```python
from build123d import *

# Parameters (mm, degrees)
SKETCH1_R           = 11.2
BOSS_EXTRUDE1_DEPTH = 50.8
SKETCH2_R           = 3.675
CUT_EXTRUDE1_DEPTH  = 50.8


with BuildPart() as part:
    # Sketch1 → Boss-Extrude1 (new body)
    with BuildSketch(Plane.XY):
        with BuildLine():
            Line((-25.4, -36.364999962), (-25.4, 36.365))
            ThreePointArc((-25.4, 36.365), (-23.726115254, 40.406115254), (-19.685, 42.08))
            Line((-19.685, 42.08), (32.385, 42.08))
            ThreePointArc((32.385, 42.08), (36.426115254, 40.406115254), (38.1, 36.365))
            Line((38.1, 36.365), (38.1, 35.095))
            ThreePointArc((38.1, 35.095), (36.426115254, 31.053884746), (32.385, 29.38))
            Line((32.385, 29.38), (-9.652, 29.38))
            ThreePointArc((-9.652, 29.38), (-11.807261469, 28.487261469), (-12.7, 26.332))
            Line((-12.7, 26.332), (-12.7, 22.503))
            ThreePointArc((-12.7, 22.503), (-11.807261469, 20.347738531), (-9.652, 19.455))
            Line((-9.652, 19.455), (0, 19.455))
            Line((0, 19.455), (13.74, 19.455))
            ThreePointArc((13.74, 19.455), (17.781115254, 17.781115254), (19.455, 13.74))
            Line((19.455, 13.74), (19.455, 0))
            Line((19.455, 0), (19.455, -13.74))
            ThreePointArc((19.455, -13.74), (17.781115254, -17.781115254), (13.74, -19.455))
            Line((13.74, -19.455), (0, -19.455))
            Line((0, -19.455), (-9.652, -19.455))
            ThreePointArc((-9.652, -19.455), (-11.807261469, -20.347738531), (-12.7, -22.503))
            Line((-12.7, -22.503), (-12.7, -26.331999962))
            ThreePointArc((-12.7, -26.331999962), (-11.807261469, -28.487261431), (-9.652, -29.379999962))
            Line((-9.652, -29.379999962), (32.385, -29.379999962))
            ThreePointArc((32.385, -29.379999962), (36.426115254, -31.053884708), (38.1, -35.094999962))
            Line((38.1, -35.094999962), (38.1, -68.114999962))
            ThreePointArc((38.1, -68.114999962), (36.426115254, -72.156115216), (32.385, -73.829999962))
            Line((32.385, -73.829999962), (31.115, -73.829999962))
            ThreePointArc((31.115, -73.829999962), (27.073884746, -72.156115216), (25.4, -68.114999962))
            Line((25.4, -68.114999962), (25.4, -47.794999962))
            ThreePointArc((25.4, -47.794999962), (23.726115254, -43.753884708), (19.685, -42.079999962))
            Line((19.685, -42.079999962), (-19.685, -42.079999962))
            ThreePointArc((-19.685, -42.079999962), (-23.726115254, -40.406115216), (-25.4, -36.364999962))
        make_face()
        Circle(SKETCH1_R, mode=Mode.SUBTRACT)
    extrude(amount=BOSS_EXTRUDE1_DEPTH)

    # Sketch2 → Cut-Extrude1 (cut)
    with BuildSketch(Plane(origin=(25.4, 0, 0), x_dir=(0, 0, -1), z_dir=(1, 0, 0))):
        with Locations((-25.4, -57.954999962)):
            Circle(SKETCH2_R)
    extrude(amount=CUT_EXTRUDE1_DEPTH, mode=Mode.SUBTRACT)


solid = part.part
```
Input: part model. Units: mm. Frame: model coordinates. A direction names the side the tool comes from. Coordinates: 2 decimals unless noted, no trailing zeros. Write each loop counter-clockwise with the first axis right and the second up, starting at its lowest first coordinate (ties: lowest second). Pieces come first, ordered by that corner, then holes. Notation, with made-up numbers: (61.25, -7.75) -> (120.25, -7.75) arc R28 cw to (120.25, 27.25) -> close; hole circle Ø1 at (32.5, 27). An arc over 180 degrees is marked (long way). Write each question's results on one line, items separated by ' | '.
Item 1: Section query D-D on x = 27. Return loops of the section in (y, z) (3 decimals), plus the area to 3 significant figures.
Conclusion:
outline: (-72.081, 0) -> (-29.38, 0) -> (-29.38, 50.8) -> (-72.081, 50.8) -> close; (29.38, 0) -> (42.08, 0) -> (42.08, 50.8) -> (29.38, 50.8) -> close; hole circle Ø7.35 at (-57.955, 25.4) | area: 2,770 mm^2
Item 2: Material intervals for probe 1 along Y at (x, z) = (0, 31) (3 decimals); probe 2 along Y at (x, z) = (5, 29) (3 decimals); probe 3 along Y at (x, z) = (31.25, 25.4), sorted ascending.
Conclusion:
probe 1: y = -42.08 to -29.38, -19.455 to -11.2, 11.2 to 19.455, 29.38 to 42.08 | probe 2: y = -42.08 to -29.38, -19.455 to -10.022, 10.022 to 19.455, 29.38 to 42.08 | probe 3: y = -73.83 to -61.63, -54.28 to -29.38, 29.38 to 42.08
Item 3: Set-up query: faces 4 (the flat face through (-25.4, -1, 25)), 5 (the cylindrical face through (-11.831, -28.463, 25.044)), 6 (the flat face through (0, -42.08, 25)). Return all of +Z, -Z, +X, -X, +Y, -Y with unobstructed straight access to the full face (end or side cutting, diameter ignored); none if empty.
Conclusion:
face 4: +Z, -Z, -X, +Y, -Y | face 5: +Z, -Z, +X | face 6: +Z, -Z, -X, -Y
Item 4: Section query A-A on z = 25.4. Count the separate pieces of the cut face and the enclosed holes in it, plus the area to 3 significant figures.
Conclusion:
separate pieces: 2 | enclosed holes: 1 | area: 3,480 mm^2
Item 5: Section query B-B on x = 0. Return loops of the section in (y, z) (3 decimals).
Conclusion:
outline: (-42.08, 0) -> (-29.38, 0) -> (-29.38, 50.8) -> (-42.08, 50.8) -> close; (-19.455, 0) -> (-11.2, 0) -> (-11.2, 50.8) -> (-19.455, 50.8) -> close; (11.2, 0) -> (19.455, 0) -> (19.455, 50.8) -> (11.2, 50.8) -> close; (29.38, 0) -> (42.08, 0) -> (42.08, 50.8) -> (29.38, 50.8) -> close
Item 6: Mould query, pull axis Y, two halves, no side actions, for faces 1 (the flat face through (6, 42.08, 25)), 2 (the cylindrical face through (17.825, -17.736, 25.044)), 3 (the cylindrical face through (36.47, -72.11, 25.04)). Classes: +Y half, -Y half, draft (parallel to the pull), parting line (faces both ways), or undercut.
Conclusion:
face 1: +Y half | face 2: undercut | face 3: -Y half
Item 7: Section query C-C on y = 0. Return loops of the section in (x, z) (3 decimals), plus the area to 3 significant figures.
Conclusion:
outline: (-25.4, 0) -> (-11.2, 0) -> (-11.2, 50.8) -> (-25.4, 50.8) -> close; (11.2, 0) -> (19.455, 0) -> (19.455, 50.8) -> (11.2, 50.8) -> close | area: 1,140 mm^2
Item 8: Pin query (flat end, axial travel): pin 1 Ø21 at (x, z) = (17.5, 32.5) entering from -Y; pin 2 Ø10 at (y, z) = (-57.5, 16) entering from -X; pin 3 Ø3 at (x, y) = (11.5, -9) entering from -Z; pin 4 Ø4 at (y, z) = (23.5, 21) entering from +X. Return the tip coordinate at first contact, or that it passes through.
Conclusion:
pin 1: stops at y = -72.91 | pin 2: stops at x = 25.4 | pin 3: stops at z = 0 | pin 4: stops at x = -12.53
